from build123d import *

# Parameters (mm, degrees)
BOSS_EXTRUDE1_DEPTH = 10
FILLET1_R           = 0.5


with BuildPart() as part:
    # Sketch2 → Boss-Extrude1 (new body)
    with BuildSketch(Plane(origin=(0, 0, 0), x_dir=(1, 0, 0), z_dir=(0, 1, 0))):
        Polygon((0, 0), (8.461538462, 8.461538462), (8.461538462, 49.123931624), (34.959843123, 49.123931624), (40.27906686, 43.804707886), (27.382478632, 30.908119658), (22.063254895, 30.908119658), (16.744031157, 25.58889592), (27.382478632, 25.58889592), (40.27906686, 5.876068376), (40.27906686, 0), (50, 0), (50, 5.876068376), (34.959843123, 27.5), (50, 44.893162393), (38.311965812, 55), (0, 55), align=None)
    extrude(amount=BOSS_EXTRUDE1_DEPTH)

    # Fillet1
    fillet1_edges = [part.edges().sort_by_distance(p)[0] for p in [
        (0, 5, -55),
        (38.311965812, 5, -55),
        (50, 5, -44.893162393),
        (50, 5, -5.876068376),
        (50, 5, 0),
        (40.27906686, 5, 0),
        (16.744031157, 5, -25.58889592),
        (22.063254895, 5, -30.908119658),
        (8.461538462, 5, -8.461538462),
        (0, 5, 0),
    ]]
    fillet(fillet1_edges, radius=FILLET1_R)


solid = part.part
The listing builds one solid part. Answer for the finished solid, in the listing's coordinates (mm). A direction names the side the tool comes from. Give positions to 0.01 mm unless a question says otherwise; leave off trailing zeros. Write each loop counter-clockwise with the first axis right and the second up, starting at its lowest first coordinate (ties: lowest second). Pieces come first, ordered by that corner, then holes.
1) Given P1, Ø3, axis at x = 8, z = -5.5, coming from the +Y side, flat-ended and moving along its own axis, determine where the tip first touches the part or whether it passes through.
2) Section C-C (y = 8.75) is taken. Write down the section's boundary in (x, z), and give its area (3 significant figures).
3) Find the intervals of material crossed by L1, parallel to Z at x = 38.5, y = 1.75; L2, parallel to Z at x = 36, y = 9; L3, parallel to Z at x = 24, y = 1, in increasing order.
4) For a pull along Z with two mould halves and no side action, classify faces 5 (the face through (23, 5, -25.589)), 6 (the face through (8.462, 5, -29)), 7 (the face through (22, 5, -49.124)) as pulls with the +Z half, pulls with the -Z half, needs draft (parallel to the pull), parting line crosses it, or undercut.
5) Section D-D (x = 11) is taken. Write down the section's boundary in (y, z).
6) Section A-A (x = 26.5) is taken. Write down the section's boundary in (y, z).
7) Section B-B (z = -4.5) is taken. Write down the section's boundary in (x, y).
8) A tool of negligible diameter and unlimited length cuts with its end or side. For faces 1 (the face through (37.582, 4.93, -46.502)), 2 (the face through (45, 5, 0)), 3 (the face through (5, 5, -5)), 4 (the face through (42.213, 4.93, -35.888)), from which of +Z, -Z, +X, -X, +Y, -Y can it reach the whole face along a straight path? Write none if from no direction.
Response:
1. P1: passes through
2. outline: (0, -54.5) arc R0.5 ccw to (0.5, -55) - (38.13, -55) arc R0.5 ccw to (38.45, -54.88) - (49.62, -45.22) arc R0.5 ccw to (49.67, -44.51) - (34.96, -27.5) - (49.91, -6) arc R0.5 ccw to (50, -5.72) - (50, -0.5) arc R0.5 ccw to (49.5, 0) - (40.78, 0) arc R0.5 ccw to (40.28, -0.5) - (40.28, -5.88) - (27.38, -25.59) - (17.95, -25.59) arc R0.5 ccw to (17.6, -26.44) - (21.92, -30.76) arc R0.5 ccw to (22.27, -30.91) - (27.38, -30.91) - (40.28, -43.8) - (34.96, -49.12) - (8.46, -49.12) - (8.46, -8.67) arc R0.5 ccw to (8.32, -8.32) - (0.85, -0.85) arc R0.5 ccw to (0, -1.21) - close
2. area: 1,130 mm2
3. L1: z = -54.84 to -45.58, -42.03 to -31.59, -22.41 to -8.6
3. L2: z = -55 to -48.08, -39.53 to -28.7, -26 to -12.42
3. L3: z = -55 to -49.12, -30.91 to -25.59
4. face 5: pulls with the +Z half
4. face 6: needs draft
4. face 7: undercut
5. outline: (0, -55) - (10, -55) - (10, -49.12) - (0, -49.12) - close
6. outline: (0, -55) - (10, -55) - (10, -49.12) - (0, -49.12) - close; (0, -30.91) - (10, -30.91) - (10, -25.59) - (0, -25.59) - close
7. outline: (0, 0) - (4.5, 0) - (4.5, 10) - (0, 10) - close; (40.28, 0) - (50, 0) - (50, 10) - (40.28, 10) - close
8. face 1: +Y, -Y
8. face 2: +Z, +X, -X, +Y, -Y
8. face 3: +Z, +Y, -Y
8. face 4: +X, +Y, -Y
